from build123d import *

# Parameters (mm, degrees)
SKETCH1_R           = 14
BOSS_EXTRUDE1_DEPTH = 18
SKETCH2_R           = 11
SKETCH3_R           = 3
SKETCH3_R_2         = 1.5
BOSS_EXTRUDE2_DEPTH = 1
SKETCH4_R           = 2
BOSS_EXTRUDE3_DEPTH = 10.5
SKETCH7_R           = 14
BOSS_EXTRUDE5_DEPTH = 2
SKETCH5_R           = 9
SKETCH6_R           = 4.5
BOSS_EXTRUDE4_DEPTH = 2
SKETCH9_R           = 1.5
CUT_EXTRUDE5_DEPTH  = 4
SKETCH10_R          = 1.5
CUT_EXTRUDE6_DEPTH  = 4
SKETCH11_R          = 1
CUT_EXTRUDE7_DEPTH  = 2
CUT_EXTRUDE8_DEPTH  = 4
SKETCH13_R          = 11.5
CUT_EXTRUDE9_DEPTH  = 22.5
FILLET1_R           = 0.5


with BuildPart() as part:
    # Sketch1 → Boss-Extrude1 (new body)
    with BuildSketch(Plane(origin=(0, 0, 0), x_dir=(1, 0, 0), z_dir=(0, 1, 0))):
        Circle(SKETCH1_R)
    extrude(amount=BOSS_EXTRUDE1_DEPTH)

    # Sketch2 → section 0 of loft1
    with BuildSketch(Plane(origin=(0, 25, 0), x_dir=(1, 0, 0), z_dir=(0, 1, 0)), mode=Mode.PRIVATE) as loft1_s0:
        Circle(SKETCH2_R)
    # loft up to a face of the part (loft1)
    loft([loft1_s0.sketch, part.faces().sort_by_distance((0, 18, 0))[0]])

    # Sketch3 → Boss-Extrude2 (add)
    with BuildSketch(Plane(origin=(0, 25, 0), x_dir=(1, 0, 0), z_dir=(0, 1, 0))):
        Circle(SKETCH3_R)
        Circle(SKETCH3_R_2, mode=Mode.SUBTRACT)
    extrude(amount=BOSS_EXTRUDE2_DEPTH)

    # Sketch4 → Boss-Extrude3 (add)
    with BuildSketch(Plane(origin=(0, 25, 0), x_dir=(1, 0, 0), z_dir=(0, 1, 0))):
        Circle(SKETCH4_R)
    extrude(amount=BOSS_EXTRUDE3_DEPTH)

    # Sketch7 → Boss-Extrude5 (add)
    with BuildSketch(Plane.XZ):
        Circle(SKETCH7_R)
    extrude(amount=BOSS_EXTRUDE5_DEPTH)

    # Sketch5 → section 0 of loft2
    with BuildSketch(Plane(origin=(0, -6, 0), x_dir=(-1, 0, 0), z_dir=(0, -1, 0)), mode=Mode.PRIVATE) as loft2_s0:
        Circle(SKETCH5_R)
    # loft up to a face of the part (loft2)
    loft([loft2_s0.sketch, part.faces().sort_by_distance((0, -2, 0))[0]])

    # Sketch6 → Boss-Extrude4 (add)
    with BuildSketch(Plane.XZ.offset(6)):
        Circle(SKETCH6_R)
    extrude(amount=BOSS_EXTRUDE4_DEPTH)

    # Sketch9 → Cut-Extrude5 (cut)
    with BuildSketch(Plane(origin=(0, 25, 0), x_dir=(1, 0, 0), z_dir=(0, 1, 0))):
        with Locations((0, 9)):
            Circle(SKETCH9_R)
        with Locations((9, 0)):
            Circle(SKETCH9_R)
        with Locations((0, -9)):
            Circle(SKETCH9_R)
        with Locations((-9, 0)):
            Circle(SKETCH9_R)
    extrude(amount=-CUT_EXTRUDE5_DEPTH, mode=Mode.SUBTRACT)

    # Sketch10 → Cut-Extrude6 (cut)
    with BuildSketch(Plane.XZ.offset(6)):
        with Locations((0, 9)):
            Circle(SKETCH10_R)
        with Locations((9, 0)):
            Circle(SKETCH10_R)
        with Locations((0, -9)):
            Circle(SKETCH10_R)
        with Locations((-9, 0)):
            Circle(SKETCH10_R)
    extrude(amount=-CUT_EXTRUDE6_DEPTH, mode=Mode.SUBTRACT)

    # Sketch11 → Cut-Extrude7 (cut)
    with BuildSketch(Plane.XZ.offset(6)):
        with Locations((0, 6)):
            Circle(SKETCH11_R)
        with Locations((6, 0)):
            Circle(SKETCH11_R)
        with Locations((0, -6)):
            Circle(SKETCH11_R)
        with Locations((-6, 0)):
            Circle(SKETCH11_R)
    extrude(amount=-CUT_EXTRUDE7_DEPTH, mode=Mode.SUBTRACT)

    # Sketch12 → Cut-Extrude8 (cut)
    with BuildSketch(Plane(origin=(0, 25, 0), x_dir=(1, 0, 0), z_dir=(0, 1, 0))):
        with BuildLine():
            Line((-10.242019056, -4.012610829), (-13.01419905, -6.784790823))
            Line((-13.01419905, -6.784790823), (-6.784790823, -13.01419905))
            Line((-6.784790823, -13.01419905), (-4.012610829, -10.242019056))
            ThreePointArc((-4.012610829, -10.242019056), (-4.596194078, -4.596194078), (-10.242019056, -4.012610829))
        make_face()
        with BuildLine():
            Line((-13.01419905, 6.784790823), (-10.242019056, 4.012610829))
            ThreePointArc((-10.242019056, 4.012610829), (-4.596194078, 4.596194078), (-4.012610829, 10.242019056))
            Line((-4.012610829, 10.242019056), (-6.784790823, 13.01419905))
            Line((-6.784790823, 13.01419905), (-13.01419905, 6.784790823))
        make_face()
        with BuildLine():
            Line((6.784790823, 13.01419905), (4.012610829, 10.242019056))
            ThreePointArc((4.012610829, 10.242019056), (4.596194078, 4.596194078), (10.242019056, 4.012610829))
            Line((10.242019056, 4.012610829), (13.01419905, 6.784790823))
            Line((13.01419905, 6.784790823), (6.784790823, 13.01419905))
        make_face()
        with BuildLine():
            Line((13.01419905, -6.784790823), (10.242019056, -4.012610829))
            ThreePointArc((10.242019056, -4.012610829), (4.596194078, -4.596194078), (4.012610829, -10.242019056))
            Line((4.012610829, -10.242019056), (6.784790823, -13.01419905))
            Line((6.784790823, -13.01419905), (13.01419905, -6.784790823))
        make_face()
    extrude(amount=-CUT_EXTRUDE8_DEPTH, mode=Mode.SUBTRACT)

    # Sketch13 → Cut-Extrude9 (cut)
    with BuildSketch(Plane(origin=(0, 21, 0), x_dir=(1, 0, 0), z_dir=(0, 1, 0))):
        Circle(SKETCH13_R)
    extrude(amount=-CUT_EXTRUDE9_DEPTH, mode=Mode.SUBTRACT)

    # Fillet1
    fillet1_edges = [part.edges().sort_by_distance(p)[0] for p in [
        (-2, 35.5, 0),
        (-4.5, -8, 0),
    ]]
    fillet(fillet1_edges, radius=FILLET1_R)

    # Sketch17 → Cut-Revolve1 (revolve, cut)
    with BuildSketch(Plane.XY):
        Polygon((-10.36813992, 23.5), (-11.439568492, 21), (-5, 21), (-5, 23.5), align=None)
    revolve(axis=Axis((0, 25, 0), (0, -1, 0)), mode=Mode.SUBTRACT)


solid = part.part
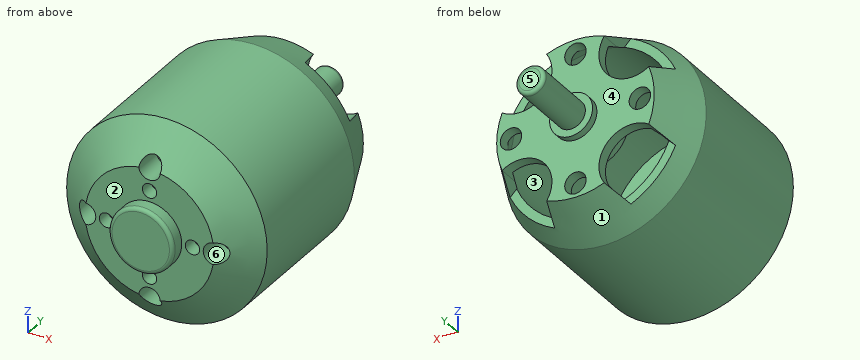
Here's how the part is built. I have some questions about the finished solid (model axes, mm). Face numbers are marked on the shaded views. A direction names the side the tool comes from. Give positions to 0.01 mm unless a question says otherwise; leave off trailing zeros. Order: outer loops, then holes, each group sorted by start corner. A loop starts at its lowest first (then second) coordinate and runs counter-clockwise, first axis right, second up. Notation, with made-up numbers: M 7,8.25 L 51,8.25 A15 ccw 51,24.25 Z; hole C 6.5,20.5 d2. An arc over 180 degrees is marked long. Answer as a JSON object with one key per item and string values. Group by question number.
1) Suppose I cut it at D-D, the plane y = 20.5. Write out the boundary of the cut face in (x, z).
2) Suppose I cut it at B-B, the plane x = -8. Count the separate pieces of the cut face and the enclosed holes in it, plus the area to 3 significant figures.
3) On a 3-axis mill with a long thin cutter (end or side, diameter ignored), from which of +Z, -Z, +X, -X, +Y, -Y can I reach the whole of each face in a straight line? I mean the marked faces 4, 5 and 6. Say none if no direction works.
4) Suppose I cut it at A-A, the plane y = 8. Write out the boundary of the cut face in (x, z), plus the area to 3 significant figures.
5) Suppose I cut it at C-C, the plane y = 26.5. Write out the boundary of the cut face in (x, z), plus the area to 3 significant figures.
6) I'm going to push flat-ended pins straight in: pin 1 Ø1 at (x, z) = (6, 0) entering from -Y; pin 2 Ø1.8 at (x, z) = (9, 0) entering from +Y; pin 3 Ø5 at (y, z) = (9, 9) entering from -X. Where does each tip first touch, or does it pass through?
7) Please list where these lines run through material, in increasing order: L1, parallel to Y at x = -4.5, z = -2.5; L2, parallel to Z at x = 0, y = 24; L3, parallel to Y at x = -2.5, z = 1.5. Write a range as [from, to].
8) We'd pull the mould along Y, two halves only. Please class the marked faces 1, 2 and 3: pulls with the +Y half, pulls with the -Y half, needs draft (parallel to the pull), parting line crosses it, or undercut.
Results found:
{
 "1": {"outline": "C 0,0 d25.86; hole C 0,0 d23"},
 "2": {"separate pieces": "3", "enclosed holes": "0", "area": "215 mm²"},
 "3": {"face 4": "+Y", "face 5": "+Z, -Z, +X, -X, +Y", "face 6": "-Y"},
 "4": {"outline": "C 0,0 d28; hole C 0,0 d23", "area": "200 mm²"},
 "5": {"outline": "C 0,0 d4", "area": "12.6 mm²"},
 "6": {"pin 1": "y = -4", "pin 2": "y = -1.5", "pin 3": "x = -12.4"},
 "7": {"L1": "[-6, -1.5], [23.5, 25]", "L2": "[-11.43, -10.5], [-7.5, 7.5], [10.5, 11.43]", "L3": "[-8, -1.5], [21, 26]"},
 "8": {"face 1": "pulls with the +Y half", "face 2": "pulls with the -Y half", "face 3": "undercut"}
}
